Can you work these out from the model? Positions are in its coordinate system, mm. A direction names the side the tool comes from. Give positions to 0.01 mm unless a question says otherwise; leave off trailing zeros. Order: outer loops, then holes, each group sorted by start corner. A loop starts at its lowest first (then second) coordinate and runs counter-clockwise, first axis right, second up. Notation, with made-up numbers: (88.5, 19) - (110.5, 19) arc R23 cw to (110.5, 56) - close; hole circle Ø11 at (79.5, 37.5). An arc over 180 degrees is marked (long way). One line per question, with ' | ' between items.
```python
from build123d import *

# Parameters (mm, degrees)
F0_R     = 9.525
F0_R_2   = 12.7
F0_R_3   = 6.35
F1_DEPTH = 6.35
F2_R     = 12.7
F3_R     = 4.7625
F4_R     = 6.34999
F5_DEPTH = 38.1


# Not quite as in the source:
# - a fillet or chamfer is up to 0.001 mm smaller than in the source, because OpenCascade refuses the exact size


with BuildPart() as f1:
    # F0 (on Front) → F1 (new body, symmetric)
    with BuildSketch(Plane.XZ):
        with BuildLine():
            Line((-19.05, -60.325), (-19.05, -47.625))
            ThreePointArc((-19.05, -47.625), (0, -28.575), (19.05, -47.625))
            Line((19.05, -47.625), (19.05, -60.325))
            Line((19.05, -60.325), (44.45, -60.325))
            Line((44.45, -60.325), (44.45, -43.8458790377))
            ThreePointArc((44.45, -43.8458790377), (46.1544838519, -38.4084943559), (50.6579059691, -34.9171326425))
            Line((50.6579059691, -34.9171326425), (82.0025655956, -34.9171326425))
            ThreePointArc((82.0025655956, -34.9171326425), (101.6, -15.875), (82.0025655956, 3.1671326425))
            Line((82.0025655956, 3.1671326425), (82.55, 34.925))
            ThreePointArc((82.55, 34.925), (50.8, 66.675), (19.05, 34.925))
            Line((19.05, 34.925), (19.05, 28.575))
            Line((19.05, 28.575), (-19.05, 28.575))
            Line((-19.05, 28.575), (-19.05, 34.925))
            ThreePointArc((-19.05, 34.925), (-50.8, 66.675), (-82.55, 34.925))
            Line((-82.55, 34.925), (-82.0025655956, 3.1671326425))
            ThreePointArc((-82.0025655956, 3.1671326425), (-101.6, -15.875), (-82.0025655956, -34.9171326425))
            Line((-82.0025655956, -34.9171326425), (-50.6579059691, -34.9171326425))
            ThreePointArc((-50.6579059691, -34.9171326425), (-46.1544838519, -38.4084943559), (-44.45, -43.8458790377))
            Line((-44.45, -43.8458790377), (-44.45, -60.325))
            Line((-44.45, -60.325), (-19.05, -60.325))
        make_face()
        with Locations((-82.55, -15.875)):
            Circle(F0_R, mode=Mode.SUBTRACT)
        Circle(F0_R_2, mode=Mode.SUBTRACT)
        with Locations((82.55, -15.875)):
            Circle(F0_R, mode=Mode.SUBTRACT)
        with Locations((-50.8, 34.925)):
            Circle(F0_R_2, mode=Mode.SUBTRACT)
        with Locations((50.8, 34.925)):
            Circle(F0_R_2, mode=Mode.SUBTRACT)
        with Locations((-82.55, -15.875)):
            Circle(F0_R)
        with Locations((-82.55, -15.875)):
            Circle(F0_R_3, mode=Mode.SUBTRACT)
        with Locations((82.55, -15.875)):
            Circle(F0_R)
        with Locations((82.55, -15.875)):
            Circle(F0_R_3, mode=Mode.SUBTRACT)
    extrude(amount=F1_DEPTH, both=True)

    # F2
    f2_edges = [f1.edges().sort_by_distance(p)[0] for p in [
        (-44.45, 0, -60.325),
        (44.45, 0, -60.325),
    ]]
    fillet(f2_edges, radius=F2_R)

    # F3
    f3_edges = [f1.edges().sort_by_distance(p)[0] for p in [
        (-82.002566, 0, 3.167133),
        (82.002566, 0, 3.167133),
    ]]
    fillet(f3_edges, radius=F3_R)

    # F4 (radius 6.35 in the source; OpenCascade refuses exactly that, so slightly less here)
    f4_edges = [f1.edges().sort_by_distance(p)[0] for p in [
        (-19.05, 0, 28.575),
        (19.05, 0, 28.575),
    ]]
    fillet(f4_edges, radius=F4_R)

    # F0 (on Front) → F5 (join)
    with BuildSketch(Plane.XZ):
        with Locations((-82.55, -15.875)):
            Circle(F0_R)
        with Locations((-82.55, -15.875)):
            Circle(F0_R_3, mode=Mode.SUBTRACT)
        with Locations((82.55, -15.875)):
            Circle(F0_R)
        with Locations((82.55, -15.875)):
            Circle(F0_R_3, mode=Mode.SUBTRACT)
    extrude(amount=-F5_DEPTH)


solid = f1.part
```
(1) Imagine slicing it at B-B (z = -41.5). List the corners of the cut face in (x, y) for me.
Answer below:
outline: (-44.74, -6.35) - (-18.04, -6.35) - (-18.04, 6.35) - (-44.74, 6.35) - close; (18.04, -6.35) - (44.74, -6.35) - (44.74, 6.35) - (18.04, 6.35) - close
(2) If I drill on line 1 (Z direction, x = 0, y = 0) (3 decimals); line 2 (Z direction, x = -50.8, y = -1.75) (3 decimals); line 3 (X direction, y = 15, z = -23), over which ranges is the centre line in solid material (lowest first)?
Answer below:
line 1: -28.575 to -12.7, 12.7 to 28.575 | line 2: -34.917 to 22.225, 47.625 to 66.675 | line 3: -88.87 to -76.23, 76.23 to 88.87
(3) If we mould it in two halves opening along Z, with no side actions, what happens to faces 1 (the face through (89, 38.1, -18)), 2 (the face through (101.45, -0.09, -18.27)), 3 (the face through (-2.75, 0.09, -12.4)), 4 (the face through (17.14, 0.089, 30.386))? For each: released by +Z, released by -Z, zero draft, split by the parting line, or undercut.
Answer below:
face 1: zero draft | face 2: split by the parting line | face 3: undercut | face 4: released by +Z
(4) Will these pins go through, and if not, where does the flat tip stop? pin 1 (4 mm diameter, centred on x = 0, y = -1.5, fed in from +Z) (3 decimals); pin 2 (6.5 mm diameter, centred on x = 67.5, y = -2.5, fed in from -Z); pin 3 (4 mm diameter, centred on y = -1, z = -45.5, fed in from +X).
Answer below:
pin 1: z = 28.575 | pin 2: z = -34.92 | pin 3: x = 44.46
(5) Imagine slicing it at A-A (x = -1). List the corners of the cut face in (y, z) for me (3 decimals), and give its area (3 significant figures).
Answer below:
outline: (-6.35, -28.601) - (6.35, -28.601) - (6.35, -12.661) - (-6.35, -12.661) - close; (-6.35, 12.661) - (6.35, 12.661) - (6.35, 28.575) - (-6.35, 28.575) - close | area: 405 mm^2
(6) Imagine slicing it at C-C (y = -3). Count the separate pieces of the cut face and the enclosed holes in it, and give its area (3 significant figures).
Answer below:
separate pieces: 1 | enclosed holes: 5 | area: 15,000 mm^2
(7) Imagine slicing it at D-D (z = 42.5). List the corners of the cut face in (x, y) for me, and give its area (3 significant figures).
Answer below:
outline: (-81.63, -6.35) - (-60.99, -6.35) - (-60.99, 6.35) - (-81.63, 6.35) - close; (-40.61, -6.35) - (-19.97, -6.35) - (-19.97, 6.35) - (-40.61, 6.35) - close; (19.97, -6.35) - (40.61, -6.35) - (40.61, 6.35) - (19.97, 6.35) - close; (60.99, -6.35) - (81.63, -6.35) - (81.63, 6.35) - (60.99, 6.35) - close | area: 1,050 mm^2
(8) On a 3-axis mill with a long thin cutter (end or side, diameter ignored), from which of +Z, -Z, +X, -X, +Y, -Y can I reach the whole of each face in a straight line? I mean faces 5 (the face through (66, 0, -34.917)), 6 (the face through (83.19, -0.09, 4.49)), 7 (the face through (-73.465, 22.003, -13.014)), 8 (the face through (0, 0, 28.575)). Say none if no direction works.
Answer below:
face 5: -Z, +X, +Y, -Y | face 6: +X, +Y, -Y | face 7: +Y | face 8: +Z, +Y, -Y
